from build123d import *

# Parameters (mm, degrees)
CROQUIS1_W              = 50
CROQUIS1_H              = 50
CROQUIS1_R              = 2
SALIENTE_EXTRUIR2_DEPTH = 0.8
CROQUIS4_R              = 4
CROQUIS4_W              = 3.55
CROQUIS4_H              = 40
CORTAR_EXTRUIR1_DEPTH   = 10
CORTAR_EXTRUIR2_START   = -39.374993
CROQUIS7_R              = 2
CORTAR_EXTRUIR2_DEPTH   = 28.749989
SALIENTE_EXTRUIR4_DEPTH = 10


with BuildPart() as part:
    # Croquis1 → Saliente-Extruir2 (new body)
    with BuildSketch(Plane.XY):
        Rectangle(CROQUIS1_W, CROQUIS1_H)
        Circle(CROQUIS1_R, mode=Mode.SUBTRACT)
    extrude(amount=SALIENTE_EXTRUIR2_DEPTH)

    # Croquis2 → Revolución1 (revolve)
    with BuildSketch(Plane(origin=(0, 0, 0), x_dir=(0, 0, -1), z_dir=(1, 0, 0))):
        Polygon((-0.8, 0), (-10.8, 0), (-10.8, 10), (-2.8, 15), (-0.8, 15), align=None)
    revolve(axis=Axis((0, 0, 0.8), (0, 0, 1)))

    # Croquis4 → Cortar-Extruir1 (cut)
    with BuildSketch(Plane.XY.offset(10.8)):
        Circle(CROQUIS4_R)
        with Locations((-6.675, 0)):
            Rectangle(CROQUIS4_W, CROQUIS4_H)
        with Locations((6.675, 0)):
            Rectangle(CROQUIS4_W, CROQUIS4_H)
    extrude(amount=-CORTAR_EXTRUIR1_DEPTH, mode=Mode.SUBTRACT)

    # Croquis7 → Cortar-Extruir2 (cut)
    with BuildSketch(Plane.ZY.offset(25).offset(CORTAR_EXTRUIR2_START)):
        with Locations((5.8, 0)):
            Circle(CROQUIS7_R)
    extrude(amount=CORTAR_EXTRUIR2_DEPTH, mode=Mode.SUBTRACT)

    # Croquis3 → Saliente-Extruir4 (add)
    with BuildSketch(Plane.XY.offset(0.8)):
        with BuildLine():
            Line((20, -25), (25, -25))
            Line((25, -25), (25, -20))
            ThreePointArc((25, -20), (28.535533906, -28.535533906), (20, -25))
        make_face()
    extrude(amount=SALIENTE_EXTRUIR4_DEPTH)


with BuildPart() as saliente_extruir4_kept_piece:
    # of the separate pieces the step leaves, the one the design keeps (saliente_extruir4_pieces_kept)
    add(part.part.solids().sort_by_distance((25, -25, 0))[0])


solid = saliente_extruir4_kept_piece.part
Read the model definition and answer for the solid it produces. Units are mm, in the model's axes. A direction names the side the tool comes from. Give positions to 0.01 mm unless a question says otherwise; leave off trailing zeros. Write each loop counter-clockwise with the first axis right and the second up, starting at its lowest first coordinate (ties: lowest second). Pieces come first, ordered by that corner, then holes. Notation, with made-up numbers: (-11.75, 38.5) - (-0.75, 38.5) arc R26 ccw to (-0.75, 69.5) - close; hole circle Ø6 at (-24, -4.75). An arc over 180 degrees is marked (long way). Use CSV: the item, a comma, the result in double quotes. Start each with the question number.
(1) For faces 4 (the flat face through (-8.45, -0.2, 3.6)), 5 (the cylindrical face through (-15, 0, 2)), 6 (the cylindrical face through (0, -15, 2)), determine the directions among +Z, -Z, +X, -X, +Y, -Y from which every point of the face is accessible in a straight line to the end or side of a thin tool.
(2) Determine the mould class of faces 1 (the conical face through (-0.09, -12.535, 6.744)), 2 (the cylindrical face through (10.796, 0.088, 3.802)), 3 (the flat face through (8.45, -0.2, 3.6)) for opening direction X: +X half, -X half, draft (parallel to the pull), parting line (faces both ways), or undercut.
(3) Consider line 1 along Y through (x, z) = (0, 0.65); line 2 along X through (y, z) = (5, 1); line 3 along X through (y, z) = (-9, 4.5). Determine where each line is inside the solid, lowest interval first.
(4) Given P1, Ø1.5, axis at x = -19.5, y = -15.5, coming from the +Z side; P2, Ø5, axis at y = 0, z = 5.8, coming from the +X side; P3, Ø5, axis at y = 5, z = 8, coming from the +X side, each flat-ended and moving along its own axis, determine where each tip first touches the part or whether it passes through.
(5) Find section C-C (y = 18.5). Give the vertices of the cut face in (x, z).
(6) Find section A-A (x = 0). Give the vertices of the cut face in (y, z).
(7) Find section B-B (z = 5.8). Give the vertices of the cut face in (x, y) (3 decimals), plus the area to 3 significant figures.
Findings below:
1,face 4,"+Z, +Y, -Y"
1,face 5,"+Z, -X"
1,face 6,"+Z, -Y"
2,face 1,"parting line"
2,face 2,"draft"
2,face 3,"undercut"
3,line 1,"-25 to -2, 2 to 25"
3,line 2,"-14.14 to -8.45, -4.9 to 4.9, 8.45 to 14.14"
3,line 3,"-10.64 to -8.45, -4.9 to 4.9, 8.45 to 10.64"
4,P1,"z = 0.8"
4,P2,"x = 14.69"
4,P3,"x = 12.56"
5,outline,"(-25, 0) - (25, 0) - (25, 0.8) - (-25, 0.8) - close"
6,outline,"(-25, 0) - (-2, 0) - (-2, 0.8) - (-4, 0.8) - (-4, 10.8) - (-10, 10.8) - (-15, 2.8) - (-15, 0.8) - (-25, 0.8) - close; (2, 0) - (25, 0) - (25, 0.8) - (15, 0.8) - (15, 2.8) - (10, 10.8) - (4, 10.8) - (4, 0.8) - (2, 0.8) - close"
7,outline,"(-12.972, -2) arc R13.125 ccw to (-8.45, -10.043) - (-8.45, -2) - close; (-12.972, 2) - (-8.45, 2) - (-8.45, 10.043) arc R13.125 ccw to start; (-4.9, -12.176) arc R13.125 ccw to (4.9, -12.176) - (4.9, -2) - (3.464, -2) arc R4 cw to (-3.464, -2) - (-4.9, -2) - close; (-4.9, 2) - (-3.464, 2) arc R4 cw to (3.464, 2) - (4.9, 2) - (4.9, 12.176) arc R13.125 ccw to (-4.9, 12.176) - close; (8.45, -10.043) arc R13.125 ccw to (12.972, -2) - (8.45, -2) - close; (8.45, 2) - (12.972, 2) arc R13.125 ccw to (8.45, 10.043) - close"
7,area,"286 mm2"
